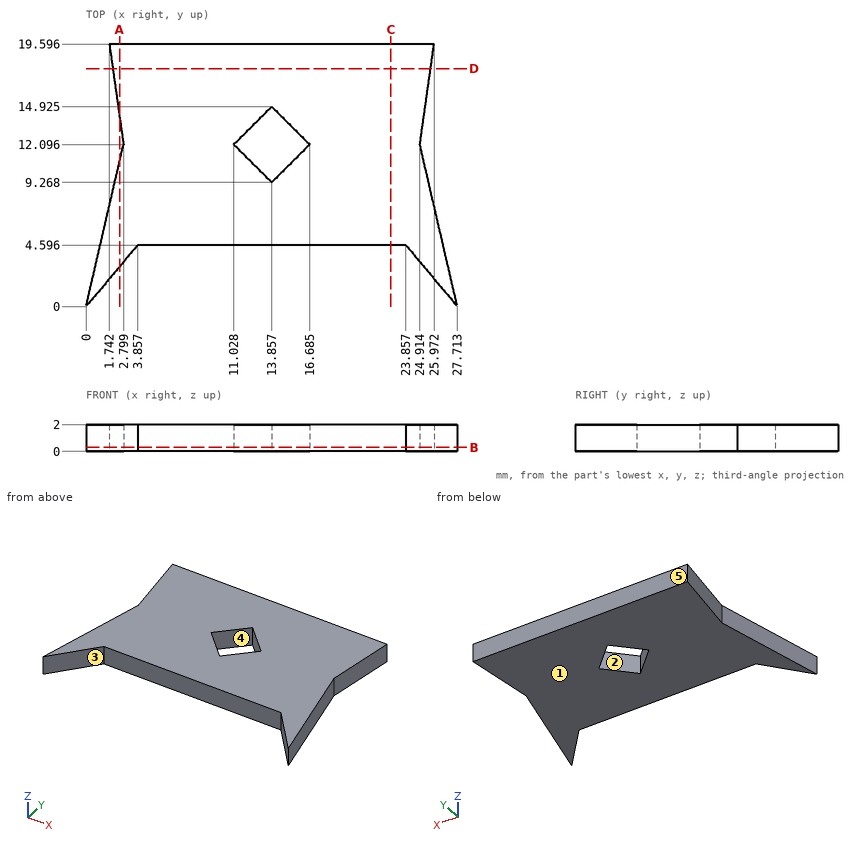
Geometry check sheet. Reference: drawing and pictorial views, mm from the part's lowest x, y, z. A direction names the side the tool comes from. Coordinates: 2 decimals unless noted, no trailing zeros. Order: outer loops, then holes, each group sorted by start corner. A loop starts at its lowest first (then second) coordinate and runs counter-clockwise, first axis right, second up.
Item 1: Section check B-B, the plane z = 0.3. Enter the section's corners in (x, y) (1 decimal).
Filled in:
outline: (0, 0) - (3.9, 4.6) - (23.9, 4.6) - (27.7, 0) - (24.9, 12.1) - (26, 19.6) - (1.7, 19.6) - (2.8, 12.1) - close; hole (11, 12.1) - (13.9, 9.3) - (16.7, 12.1) - (13.9, 14.9) - close
Item 2: Section check A-A, the plane x = 2.5. Enter the section's corners in (y, z), then the cut area to 3 significant figures.
Filled in:
outline: (2.98, 0) - (10.8, 0) - (10.8, 2) - (2.98, 2) - close; (14.22, 0) - (19.6, 0) - (19.6, 2) - (14.22, 2) - close
area: 26.4 mm2
Item 3: Section check C-C, the plane x = 22.75. Enter the section's corners in (y, z), then the cut area to 3 significant figures.
Filled in:
outline: (4.6, 0) - (19.6, 0) - (19.6, 2) - (4.6, 2) - close
area: 30.0 mm2
Item 4: Release check for a two-part mould opening along X. For the marked faces 4 and 5 record: +X half, -X half, draft (parallel to the pull), parting line (faces both ways), or undercut.
Filled in:
face 4: undercut
face 5: draft
Item 5: Material ranges on L1, parallel to Y at x = 8, z = 1.05; L2, parallel to X at y = 1.5, z = 0.5 (1 decimal); L3, parallel to X at y = 9.75, z = 1.55 (1 decimal), recorded low to high.
Filled in:
L1: y = 4.6 to 19.6
L2: x = 0.3 to 1.3, 26.5 to 27.4
L3: x = 2.3 to 13.4, 14.3 to 25.5
Item 6: Access from +Z, -Z, +X, -X, +Y, -Y to the whole of each face (thin tool, end or side, straight path). Record for the marked faces 1, 2 and 3.
Filled in:
face 1: -Z, +X, -X, +Y, -Y
face 2: +Z, -Z
face 3: +Z, -Z, -Y
Item 7: Section check D-D, the plane y = 17.75. Enter the section's corners in (x, z).
Filled in:
outline: (2, 0) - (25.71, 0) - (25.71, 2) - (2, 2) - close
